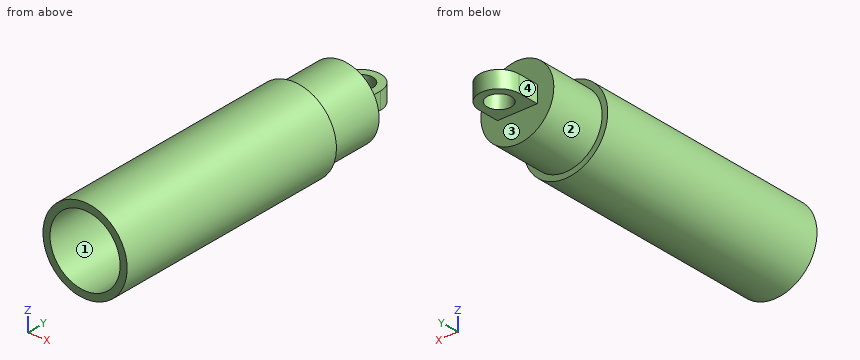
from build123d import *

# Parameters (mm, degrees)
SKETCH_1_R               = 9
EXTRUDE_1_DEPTH          = 52
SKETCH_2_R               = 7.8
EXTRUDE_2_DEPTH          = 12
EXTRUDE_3_DEPTH          = 1.8
EXTRUDE_3_DEPTH_BACK     = 1.8
SKETCH_3_R               = 2.6
EXTRUDE_4_DEPTH          = 1.8
EXTRUDE_4_DEPTH_BACK     = 1.8
SKETCH_4_R               = 1.6
CUT_EXTRUDE_1_DEPTH      = 27
CUT_EXTRUDE_1_DEPTH_BACK = 36
SKETCH_5_R               = 7.5


with BuildPart() as part:
    # Sketch 1 → Extrude 1 (new body)
    with BuildSketch(Plane(origin=(0, 0, 0), x_dir=(1, 0, 0), z_dir=(0, 1, 0))):
        with Locations(Location((0, 0, 0), (0, 0, 90))):
            Circle(SKETCH_1_R)
    extrude(amount=EXTRUDE_1_DEPTH)

    # Sketch 2 → Extrude 2 (add)
    with BuildSketch(Plane(origin=(0, 52, 0), x_dir=(1, 0, 0), z_dir=(0, 1, 0))):
        with Locations(Location((0, 0, 0), (0, 0, 270))):
            Circle(SKETCH_2_R)
    extrude(amount=EXTRUDE_2_DEPTH)

    # Sketch 3 → Extrude 3 (add, two sides: drawn at the far end of the back side and taken through both)
    with BuildSketch(Plane.XY.offset(-EXTRUDE_3_DEPTH_BACK)):
        with BuildLine():
            Line((-4.255, 59.5), (4.255, 59.5))
            Line((4.255, 59.5), (4.255, 68.5))
            ThreePointArc((4.255, 68.5), (0, 72.755), (-4.255, 68.5))
            Line((-4.255, 68.5), (-4.255, 59.5))
        make_face()
        with Locations((0, 68.5)):
            Circle(SKETCH_3_R, mode=Mode.SUBTRACT)
    extrude(amount=EXTRUDE_3_DEPTH + EXTRUDE_3_DEPTH_BACK)

    # Sketch 4 → Extrude 4 (add, two sides: drawn at the far end of the back side and taken through both)
    with BuildSketch(Plane.XY.offset(-EXTRUDE_4_DEPTH_BACK)):
        with BuildLine():
            Line((-4.65, -16.5), (-4.65, -8.5))
            Line((-4.65, -8.5), (-4.65, 0))
            Line((-4.65, 0), (4.65, 0))
            Line((4.65, 0), (4.65, -8.5))
            Line((4.65, -8.5), (4.65, -16.5))
            ThreePointArc((4.65, -16.5), (0, -21.15), (-4.65, -16.5))
        make_face()
        with Locations((0, -16.5)):
            Circle(SKETCH_4_R, mode=Mode.SUBTRACT)
    extrude(amount=EXTRUDE_4_DEPTH + EXTRUDE_4_DEPTH_BACK)

    # Sketch 5 → Cut-Extrude 1 (cut, two sides: drawn at the far end of the back side and taken through both)
    with BuildSketch(Plane.XZ.offset(-CUT_EXTRUDE_1_DEPTH_BACK)):
        with Locations(Location((0, 0, 0), (0, 0, 90))):
            Circle(SKETCH_5_R)
    extrude(amount=CUT_EXTRUDE_1_DEPTH + CUT_EXTRUDE_1_DEPTH_BACK, mode=Mode.SUBTRACT)


solid = part.part
The model under review builds one solid part; all positions refer to its coordinate system, in mm. Face numbers are marked on the shaded views. Round coordinates to 2 decimals unless told otherwise and drop trailing zeros. Write each loop counter-clockwise with the first axis right and the second up, starting at its lowest first coordinate (ties: lowest second). Pieces come first, ordered by that corner, then holes. Notation, with made-up numbers: M 30.25,77 L 76.25,77 A34 cw 76.25,115 Z; hole C 38,65.5 d6. An arc over 180 degrees is marked long. Answer as CSV lines item,"result". Start each with the question number.
Q1. Consider section C-C, the plane x = 0. Give the boundary of the cut face in (y, z) (3 decimals).
Q2. Consider section A-A, the plane y = 67.5. Give the boundary of the cut face in (x, z) (3 decimals), then the cut area to 3 significant figures.
Q3. Consider section D-D, the plane x = -6. Give the boundary of the cut face in (y, z), then the cut area to 3 significant figures.
Q4. Clearance check with flat-ended pins moving along their axes: P1, Ø4.5, axis at x = 1.5, z = -3, coming from the -Y side; P2, Ø7, axis at x = -1, y = 68.5, coming from the -Z side; P3, Ø1.8, axis at y = 65.5, z = -0.5, coming from the -X side (3 decimals); P4, Ø9, axis at x = 4.5, z = 2.5, coming from the +Y side. State where each tip first meets the part, or that it passes through.
Q5. Wall thickness on line 1 along Y through (x, z) = (0, -1) (3 decimals); line 2 along X through (y, z) = (22, 0); line 3 along Y through (x, z) = (0.25, -1.5): over which ranges is each line inside the solid? List them lowest first.
Q6. Consider section B-B, the plane z = 0. Give the boundary of the cut face in (x, y) (3 decimals).
Q7. The part is to be moulded in two halves that separate along X. For the marked faces 1, 2, 3 and 4, say which applies: +X half, -X half, draft (parallel to the pull), parting line (faces both ways), or undercut.
Result set:
1,outline,"M 0,-9 L 52,-9 L 52,-7.8 L 64,-7.8 L 64,-1.8 L 65.9,-1.8 L 65.9,1.8 L 64,1.8 L 64,7.8 L 52,7.8 L 52,9 L 0,9 L 0,7.5 L 36,7.5 L 36,-7.5 L 0,-7.5 Z; M 71.1,-1.8 L 72.755,-1.8 L 72.755,1.8 L 71.1,1.8 Z"
2,outline,"M -4.255,-1.8 L -2.4,-1.8 L -2.4,1.8 L -4.255,1.8 Z; M 2.4,-1.8 L 4.255,-1.8 L 4.255,1.8 L 2.4,1.8 Z"
2,area,"13.4 mm²"
3,outline,"M 0,-6.71 L 52,-6.71 L 52,-4.98 L 64,-4.98 L 64,4.98 L 52,4.98 L 52,6.71 L 0,6.71 L 0,4.5 L 36,4.5 L 36,-4.5 L 0,-4.5 Z"
3,area,"493 mm²"
4,P1,"stops at y = 36"
4,P2,"stops at z = -1.8"
4,P3,"stops at x = -4.255"
4,P4,"stops at y = 72.75"
5,line 1,"y = 36 to 65.9, 71.1 to 72.755"
5,line 2,"x = -9 to -7.5, 7.5 to 9"
5,line 3,"y = 36 to 65.91, 71.09 to 72.75"
6,outline,"M -9,0 L -7.5,0 L -7.5,36 L 7.5,36 L 7.5,0 L 9,0 L 9,52 L 7.8,52 L 7.8,64 L 4.255,64 L 4.255,68.5 A4.255 ccw -4.255,68.5 L -4.255,64 L -7.8,64 L -7.8,52 L -9,52 Z; hole C 0,68.5 d5.2"
7,face 1,"undercut"
7,face 2,"parting line"
7,face 3,"draft"
7,face 4,"-X half"
